Check sheet for the modelled part. Datum: model origin and axes. Units: mm. A direction names the side the tool comes from. Give positions to 0.01 mm unless a question says otherwise; leave off trailing zeros. Write each loop counter-clockwise with the first axis right and the second up, starting at its lowest first coordinate (ties: lowest second). Pieces come first, ordered by that corner, then holes. Notation, with made-up numbers: M 83,25 L 140,25 A26 ccw 140,58 Z; hole C 6,32.25 d8. An arc over 180 degrees is marked long. Write item = value, one per line. Start each with the question number.
1) Cross-section at A-A, the plane y = -21.5. Record the cut outline in (x, z), plus the area to 3 significant figures.
2) Scan lines: line 1 along Y through (x, z) = (41.5, 0.75); line 2 along X through (y, z) = (32.5, 0.7); line 3 along Y through (x, z) = (-11.5, 0.3). Record each from-to range of solid material in increasing order. Write a range as [from, to].
3) Cross-section at C-C, the plane z = 1.65. Record the cut outline in (x, y), plus the area to 3 significant figures.
4) Mould release check, pull along X, two halves, no side actions. Record for faces 1 (the flat face through (-1, 36, 1)), 2 (the cylindrical face through (-39.713, -30.752, 0.493)), 3 (the flat face through (-46, -1, 1)): released by +X, released by -X, zero draft, split by the parting line, or undercut.
5) Cross-section at B-B, the plane x = 35. Record the cut outline in (y, z), plus the area to 3 significant figures.
6) Access from +Z, -Z, +X, -X, +Y, -Y to the whole of each face (thin tool, end or side, straight path). Record for faces 4 (the cylindrical face through (39.752, -30.713, 0.493)), 5 (the flat face through (-3.6, -34.5, 0)), 6 (the flat face through (-40, 31, 1)).
```python
from build123d import *

# Parameters (mm, degrees)
F0_W     = 92
F0_H     = 72
F1_DEPTH = 1
F2_W     = 92
F2_H     = 72
F2_W_2   = 90
F2_H_2   = 70
F3_DEPTH = 1.6


with BuildPart() as f1:
    # F0 (on Top) → F1 (new body)
    with BuildSketch(Plane.XY):
        Rectangle(F0_W, F0_H)
        Polygon((-41.5, 34), (-39, 34), (39, 34), (41.5, 34), (44, 34), (44, 30), (44, -30), (44, -34), (41.5, -34), (39, -34), (-39, -34), (-41.5, -34), (-44, -34), (-44, -30), (-44, 30), (-44, 34), align=None, mode=Mode.SUBTRACT)
        with BuildLine():
            Line((41.5, 34), (39, 34))
            Line((39, 34), (39, 32.5))
            ThreePointArc((39, 32.5), (39.732233, 30.732233), (41.5, 30))
            Line((41.5, 30), (44, 30))
            Line((44, 30), (44, 34))
            Line((44, 34), (41.5, 34))
        make_face()
        with BuildLine():
            ThreePointArc((43, 32.5), (40.43934, 31.43934), (41.5, 34))
            ThreePointArc((41.5, 34), (42.56066, 33.56066), (43, 32.5))
        make_face(mode=Mode.SUBTRACT)
        with BuildLine():
            Line((44, -34), (44, -30))
            Line((44, -30), (41.5, -30))
            ThreePointArc((41.5, -30), (39.732233, -30.732233), (39, -32.5))
            Line((39, -32.5), (39, -34))
            Line((39, -34), (41.5, -34))
            Line((41.5, -34), (44, -34))
        make_face()
        with BuildLine():
            ThreePointArc((43, -32.5), (42.56066, -33.56066), (41.5, -34))
            ThreePointArc((41.5, -34), (40.43934, -31.43934), (43, -32.5))
        make_face(mode=Mode.SUBTRACT)
        with BuildLine():
            Line((-41.5, -30), (-44, -30))
            Line((-44, -30), (-44, -34))
            Line((-44, -34), (-41.5, -34))
            Line((-41.5, -34), (-39, -34))
            Line((-39, -34), (-39, -32.5))
            ThreePointArc((-39, -32.5), (-39.732233, -30.732233), (-41.5, -30))
        make_face()
        with BuildLine():
            ThreePointArc((-40, -32.5), (-40.43934, -33.56066), (-41.5, -34))
            ThreePointArc((-41.5, -34), (-42.56066, -31.43934), (-40, -32.5))
        make_face(mode=Mode.SUBTRACT)
        with BuildLine():
            Line((-39, 32.5), (-39, 34))
            Line((-39, 34), (-41.5, 34))
            Line((-41.5, 34), (-44, 34))
            Line((-44, 34), (-44, 30))
            Line((-44, 30), (-41.5, 30))
            ThreePointArc((-41.5, 30), (-39.732233, 30.732233), (-39, 32.5))
        make_face()
        with BuildLine():
            ThreePointArc((-40, 32.5), (-42.56066, 31.43934), (-41.5, 34))
            ThreePointArc((-41.5, 34), (-40.43934, 33.56066), (-40, 32.5))
        make_face(mode=Mode.SUBTRACT)
    extrude(amount=F1_DEPTH)

    # F2 (on face) → F3 (join)
    with BuildSketch(Plane.XY.offset(1)):
        Rectangle(F2_W, F2_H)
        Rectangle(F2_W_2, F2_H_2, mode=Mode.SUBTRACT)
    extrude(amount=F3_DEPTH)


solid = f1.part
```
Reply:
q1.outline = M -46,0 L -44,0 L -44,1 L -45,1 L -45,2.6 L -46,2.6 Z; M 44,0 L 46,0 L 46,2.6 L 45,2.6 L 45,1 L 44,1 Z
q1.area = 7.20 mm2
q2.line_1 = [-36, -34], [-31, -30], [30, 31], [34, 36]
q2.line_2 = [-46, -43], [-40, -39], [39, 40], [43, 46]
q2.line_3 = [-36, -34], [34, 36]
q3.outline = M -46,-36 L 46,-36 L 46,36 L -46,36 Z; hole M -45,-35 L 45,-35 L 45,35 L -45,35 Z
q3.area = 324 mm2
q4.face_1 = zero draft
q4.face_2 = undercut
q4.face_3 = released by -X
q5.outline = M -36,0 L -34,0 L -34,1 L -35,1 L -35,2.6 L -36,2.6 Z; M 34,0 L 36,0 L 36,2.6 L 35,2.6 L 35,1 L 34,1 Z
q5.area = 7.20 mm2
q6.face_4 = +Z, -Z
q6.face_5 = -Z, +X, -X, +Y, -Y
q6.face_6 = +Z
